Geometry check sheet. Reference: the model listing, model coordinates, mm. Round coordinates to 2 decimals unless told otherwise and drop trailing zeros. Order: outer loops, then holes, each group sorted by start corner. A loop starts at its lowest first (then second) coordinate and runs counter-clockwise, first axis right, second up. Notation, with made-up numbers: (-12.75, -26.5) - (-8.75, -26.5) arc R26 cw to (-8.75, 1.5) - close; hole circle Ø7 at (33.5, 67.5). An arc over 180 degrees is marked (long way). Return JSON: item names as keys, results as strings. Group by question number.
Q1. Sectioned sample at D-D, the plane z = 9.25. Give the number of separate pieces and of enclosed holes in the cut face, then the cut area to 3 significant figures.
Q2. Sectioned sample at B-B, the plane x = 43. Record the cut outline in (y, z), then the cut area to 3 significant figures.
Q3. Sectioned sample at C-C, the plane y = -77. Record the cut outline in (x, z).
Q4. Sectioned sample at A-A, the plane y = -48. Record the cut outline in (x, z).
Q5. Draft check along Y on faces 1 (the cylindrical face through (153.184, -45.342, 7.465)), 2 (the flat face through (142.749, -82.757, 7.465)), 3 (the flat face through (-1, -133, 5)), 4 (the cylindrical face through (-153.11, -45.62, 7.46)). Enter one of: pulls with the +Y half, pulls with the -Y half, needs draft (parallel to the pull), parting line crosses it, or undercut.
Q6. Gauge pin test, flat ends, axial feed: pin 1 Ø2.5 at (x, y) = (0, -128.198) entering from +Z; pin 2 Ø1 at (y, z) = (-115.5, 6) entering from -X; pin 3 Ø1 at (x, z) = (-113, 5.5) entering from -Y; pin 4 Ø1.5 at (x, z) = (-35, 7) entering from +Y. Record the tip position at first contact, or that the pin passes through.
Q7. Material ranges on line 1 along Y through (x, z) = (0, 7.05); line 2 along X through (y, z) = (-1.5, 6.4); line 3 along Y through (x, z) = (-62.5, 6.3), recorded low to high.
Solid Edge part; units mm, degrees
sketch "Sketch1" plane through (0.0007, 14.651, 5) normal (0, 0, 1) x (1, 0, 0)
  line L0 (-114.0407, 98.8093) -> (-57.2599, 131.5929)
  arc A0 (-54.1474, 131.5247) -> (-57.2599, 131.5929) centre (-55.7598, 128.9948) ccw
  arc A1 (-47.0142, 137.1861) -> (-48.7662, 134.4664) centre (-45.7662, 134.458) ccw
  arc A2 (-47.0142, 137.1861) -> (-26.9146, 142.5706) centre (-21.0226, 80.3698) cw
  arc A3 (-24.0376, 141.0909) -> (-26.9146, 142.5706) centre (-26.6317, 139.5839) ccw
  arc A4 (-15.245, 142.849) -> (-17.9063, 141.2336) centre (-15.245, 139.849) ccw
  line L1 (-15.245, 142.849) -> (15.2436, 142.849)
  arc A5 (17.905, 141.2336) -> (15.2436, 142.849) centre (15.2436, 139.849) ccw
  arc A6 (26.9132, 142.5696) -> (24.036, 141.0904) centre (26.6298, 139.583) ccw
  arc A7 (26.9132, 142.5696) -> (47.0027, 137.1869) centre (21.0099, 80.3561) cw
  arc A8 (48.7549, 134.4673) -> (47.0027, 137.1869) centre (45.7549, 134.4587) ccw
  arc A9 (57.2487, 131.5943) -> (54.1362, 131.526) centre (55.7487, 128.9962) ccw
  line L2 (57.2487, 131.5943) -> (114.0299, 98.8129)
  arc A10 (115.5271, 96.0833) -> (114.0299, 98.8129) centre (112.5299, 96.2148) ccw
  arc A11 (124.0003, 92.7805) -> (120.7849, 92.9052) centre (122.2944, 90.3127) ccw
  arc A12 (124.0003, 92.7805) -> (155.0355, 39.027) centre (82.7747, 33.1424) cw
  arc A13 (153.5358, 36.1799) -> (155.0355, 39.027) centre (152.0454, 38.7835) ccw
  arc A14 (155.2747, 27.3761) -> (153.6593, 30.0375) centre (152.2747, 27.3761) ccw
  line L3 (155.2747, 27.3761) -> (155.2747, -38.192)
  arc A15 (153.6593, -40.8534) -> (155.2747, -38.192) centre (152.2747, -38.192) ccw
  arc A16 (154.9954, -49.8615) -> (153.5161, -46.9844) centre (152.0088, -49.5782) ccw
  arc A17 (154.9954, -49.8615) -> (149.6134, -69.9554) centre (92.7533, -43.9583) cw
  arc A18 (146.8942, -71.7079) -> (149.6134, -69.9554) centre (146.8851, -68.7079) ccw
  arc A19 (144.0217, -80.2016) -> (143.9534, -77.0892) centre (141.4236, -78.7016) ccw
  line L4 (144.0217, -80.2016) -> (127.6444, -108.5679)
  arc A20 (122.7007, -116.5716) -> (122.8583, -113.3403) centre (120.256, -114.8329) ccw
  arc A21 (77.6703, -142.5696) -> (122.7007, -116.5716) centre (71.767, -80.3476) ccw
  arc A22 (74.7931, -141.0904) -> (77.6703, -142.5696) centre (77.3869, -139.583) ccw
  arc A23 (66.0007, -142.849) -> (68.6621, -141.2336) centre (66.0007, -139.849) ccw
  line L5 (5.7656, -142.849) -> (66.0007, -142.849)
  arc A24 (3.1042, -141.2336) -> (5.7656, -142.849) centre (5.7656, -139.849) ccw
  arc A25 (-5.767, -142.849) -> (-3.1056, -141.2336) centre (-5.767, -139.849) ccw
  line L6 (-66.0021, -142.849) -> (-5.767, -142.849)
  arc A26 (-68.6634, -141.2336) -> (-66.0021, -142.849) centre (-66.0021, -139.849) ccw
  arc A27 (-77.6716, -142.5694) -> (-74.7944, -141.0903) centre (-77.3881, -139.5828) ccw
  arc A28 (-122.6994, -116.5717) -> (-77.6716, -142.5694) centre (-71.7665, -80.349) ccw
  arc A29 (-122.857, -113.3404) -> (-122.6994, -116.5717) centre (-120.2547, -114.833) ccw
  arc A30 (-128.7762, -106.6053) -> (-126.0465, -108.1024) centre (-126.1781, -105.1053) ccw
  line L7 (-144.0218, -80.199) -> (-128.7762, -106.6053)
  arc A31 (-143.9535, -77.0865) -> (-144.0218, -80.199) centre (-141.4237, -78.699) ccw
  arc A32 (-149.6144, -69.9531) -> (-146.8949, -71.7053) centre (-146.8862, -68.7053) ccw
  arc A33 (-154.9987, -49.8585) -> (-149.6144, -69.9531) centre (-92.7672, -43.9523) ccw
  arc A34 (-153.5196, -46.9813) -> (-154.9987, -49.8585) centre (-152.0122, -49.5751) ccw
  arc A35 (-155.2786, -38.189) -> (-153.6631, -40.8503) centre (-152.2786, -38.1889) ccw
  line L8 (-155.2818, 27.3758) -> (-155.2786, -38.189)
  arc A36 (-153.6665, 30.0373) -> (-155.2818, 27.3758) centre (-152.2818, 27.376) ccw
  arc A37 (-155.0428, 39.0267) -> (-153.5432, 36.1796) centre (-152.0527, 38.7832) ccw
  arc A38 (-124.0109, 92.7765) -> (-155.0428, 39.0267) centre (-82.7847, 33.1421) ccw
  arc A39 (-120.7955, 92.9014) -> (-124.0109, 92.7765) centre (-122.3049, 90.3088) ccw
  arc A40 (-114.0407, 98.8093) -> (-115.5378, 96.0796) centre (-112.5406, 96.2112) ccw
  arc A41 (-48.7662, 134.4664) -> (-54.1474, 131.5247) centre (-52.2662, 134.4761) cw
  arc A42 (-17.9064, 141.2336) -> (-24.0377, 141.0909) centre (-21.0113, 142.849) cw
  arc A43 (24.036, 141.0904) -> (17.905, 141.2336) centre (21.0099, 142.849) cw
  arc A44 (54.1362, 131.526) -> (48.7549, 134.4673) centre (52.2549, 134.4774) cw
  arc A45 (120.7849, 92.9052) -> (115.5271, 96.0832) centre (119.0237, 95.9298) cw
  arc A46 (153.6593, 30.0375) -> (153.5358, 36.1799) centre (155.2747, 33.1424) cw
  arc A47 (153.5161, -46.9844) -> (153.6593, -40.8534) centre (155.2747, -43.9583) cw
  arc A48 (143.9534, -77.0891) -> (146.8942, -71.7079) centre (146.9048, -75.2079) cw
  arc A49 (122.8584, -113.3404) -> (127.6444, -108.5679) centre (125.8944, -111.599) cw
  arc A50 (68.6621, -141.2336) -> (74.7931, -141.0904) centre (71.767, -142.849) cw
  arc A51 (-3.1056, -141.2336) -> (3.1042, -141.2336) centre (-0.0007, -142.849) cw
  arc A52 (-74.7944, -141.0903) -> (-68.6635, -141.2336) centre (-71.7684, -142.849) cw
  arc A53 (-126.0466, -108.1024) -> (-122.857, -113.3404) centre (-125.8931, -111.599) cw
  arc A54 (-146.8949, -71.7053) -> (-143.9536, -77.0866) centre (-146.905, -75.2053) cw
  arc A55 (-153.6632, -40.8503) -> (-153.5196, -46.9813) centre (-155.2784, -43.9553) cw
  arc A56 (-153.5432, 36.1796) -> (-153.6665, 30.0373) centre (-155.2821, 33.1421) cw
  arc A57 (-115.5377, 96.0796) -> (-120.7955, 92.9014) centre (-119.0344, 95.926) cw
  line L9 (-56.0166, 140.971) -> (-122.7845, 102.4212)
  arc A58 (-162.7821, 33.1421) -> (-122.7845, 102.4212) centre (-82.7847, 33.1421) cw
  line L10 (-162.7821, 33.1421) -> (-162.7784, -43.9553)
  arc A59 (-162.7784, -43.9553) -> (-153.4002, -78.9553) centre (-92.7784, -43.9553) ccw
  line L11 (-132.3882, -115.349) -> (-153.4002, -78.9553)
  arc A60 (-132.3882, -115.349) -> (-71.7683, -150.349) centre (-71.7665, -80.349) ccw
  line L12 (71.767, -150.349) -> (-71.7683, -150.349)
  arc A61 (71.767, -150.349) -> (132.3896, -115.349) centre (71.7678, -80.349) ccw
  line L13 (132.3896, -115.349) -> (153.4002, -78.9576)
  arc A62 (162.7747, -43.9583) -> (153.4002, -78.9576) centre (92.791, -43.9684) cw
  line L14 (162.7747, 33.1424) -> (162.7747, -43.9583)
  arc A63 (122.7736, 102.4251) -> (162.7747, 33.1424) centre (82.7747, 33.1424) cw
  line L15 (56.0045, 140.9728) -> (122.7736, 102.4251)
  arc A64 (21.0099, 150.349) -> (56.0045, 140.9728) centre (21.008, 80.349) cw
  line L16 (-21.0112, 150.349) -> (21.0099, 150.349)
  arc A65 (-32.5074, 149.4015) -> (-21.0112, 150.349) centre (-20.997, 79.961) cw
  arc A66 (-44.641, 146.2432) -> (-32.5074, 149.4015) centre (-21.0122, 80.3518) cw
  arc A67 (-56.0166, 140.971) -> (-44.641, 146.2432) centre (-21.0122, 80.3518) cw
  circle A68 centre (-71.7683, -142.849) radius 1.5
  circle A69 centre (-0.0007, -142.849) radius 1.5
  circle A70 centre (-125.893, -111.599) radius 1.5
  circle A71 centre (-146.905, -75.2053) radius 1.5
  circle A72 centre (-155.2784, -43.9553) radius 1.5
  circle A73 centre (-155.2821, 33.1421) radius 1.5
  circle A74 centre (-119.0344, 95.9261) radius 1.5
  circle A75 centre (-52.2662, 134.4761) radius 1.5
  circle A76 centre (-21.0112, 142.849) radius 1.5
  circle A77 centre (21.0099, 142.849) radius 1.5
  circle A78 centre (52.2549, 134.4774) radius 1.5
  circle A79 centre (119.0237, 95.9298) radius 1.5
  circle A80 centre (155.2747, 33.1424) radius 1.5
  circle A81 centre (155.2747, -43.9583) radius 1.5
  circle A82 centre (146.9048, -75.2079) radius 1.5
  circle A83 centre (125.8944, -111.599) radius 1.5
  circle A84 centre (71.767, -142.849) radius 1.5
extrude "ExtrudedProtrusion_7" add sketch "Sketch1" along normal blind 5
sketch "Sketch2" plane through (-0.003, 14.651, 10) normal (0, 0, 1) x (1, 0, 0)
  line L0 (-168.1883, -5.4066) -> (170.0115, -5.4066)
  line L1 (170.0115, -5.4066) -> (170.0115, 153.6029)
  line L2 (170.0115, 153.6029) -> (-168.1883, 153.6029)
  line L3 (-168.1883, 153.6029) -> (-168.1883, -5.4066)
extrude "Cutout1" cut sketch "Sketch2" against normal up to next
properties material "Polycarbonate"
Reply:
{
 "1": {"separate pieces": "1", "enclosed holes": "9", "area": "3,970 mm^2"},
 "2": {"outline": "(-135.7, 5) - (-128.2, 5) - (-128.2, 10) - (-135.7, 10) - close", "area": "37.5 mm^2"},
 "3": {"outline": "(-146.07, 5) - (-137.41, 5) - (-137.41, 10) - (-146.07, 10) - close; (137.41, 5) - (146.07, 5) - (146.07, 10) - (137.41, 10) - close"},
 "4": {"outline": "(-160.23, 5) - (-152.42, 5) - (-152.42, 10) - (-160.23, 10) - close; (152.42, 5) - (160.24, 5) - (160.24, 10) - (152.42, 10) - close"},
 "5": {"face 1": "undercut", "face 2": "pulls with the -Y half", "face 3": "needs draft", "face 4": "undercut"},
 "6": {"pin 1": "through", "pin 2": "x = -121.46", "pin 3": "y = -122.63", "pin 4": "y = -128.2"},
 "7": {"line 1": "-135.7 to -129.7, -126.7 to -124.7", "line 2": "-162.78 to -155.28, 155.28 to 162.78", "line 3": "-135.7 to -128.2"}
}
